Verification items for the finished model (mm, model axes). Round coordinates to 2 decimals unless told otherwise and drop trailing zeros. Write each loop counter-clockwise with the first axis right and the second up, starting at its lowest first coordinate (ties: lowest second). Pieces come first, ordered by that corner, then holes. Notation, with made-up numbers: (20, 83.25) -> (26, 83.25) arc R20 ccw to (26, 122.25) -> close; hole circle Ø11 at (62.25, 46.5). An arc over 180 degrees is marked (long way). Use CSV: the item, a comma, the result in double quotes.
```python
from build123d import *

# Parameters (mm, degrees)
SKETCH1_W           = 40
SKETCH1_H           = 5
BOSS_EXTRUDE1_DEPTH = 72
SKETCH2_W           = 8
SKETCH2_H           = 72
CUT_EXTRUDE1_DEPTH  = 0.75
SKETCH3_W           = 0.6
SKETCH3_H           = 0.6
BOSS_EXTRUDE2_DEPTH = 8
SKETCH4_R           = 2.6
CUT_EXTRUDE2_DEPTH  = 83.516664984
SKETCH5_W           = 8
SKETCH5_H           = 20
CUT_EXTRUDE3_DEPTH  = 83.516664984


with BuildPart() as part:
    # Sketch1 → Boss-Extrude1 (new body)
    with BuildSketch(Plane(origin=(0, 0, 0), x_dir=(1, 0, 0), z_dir=(0, 1, 0))):
        with Locations((20, 2.5)):
            Rectangle(SKETCH1_W, SKETCH1_H)
    extrude(amount=BOSS_EXTRUDE1_DEPTH)

    # Sketch2 → Cut-Extrude1 (cut)
    with BuildSketch(Plane(origin=(0, 0, -5), x_dir=(-1, 0, 0), z_dir=(0, 0, -1))):
        with Locations((-17.2, 36)):
            Rectangle(SKETCH2_W, SKETCH2_H)
    extrude(amount=-CUT_EXTRUDE1_DEPTH, mode=Mode.SUBTRACT)

    # Sketch3 → Boss-Extrude2 (add)
    with BuildSketch(Plane(origin=(13.2, 0, 0), x_dir=(0, 0, -1), z_dir=(1, 0, 0))):
        with Locations((4.55, 71.1)):
            Rectangle(SKETCH3_W, SKETCH3_H)
        with Locations((4.55, 69.1)):
            Rectangle(SKETCH3_W, SKETCH3_H)
        with Locations((4.55, 67.1)):
            Rectangle(SKETCH3_W, SKETCH3_H)
        with Locations((4.55, 65.1)):
            Rectangle(SKETCH3_W, SKETCH3_H)
        with Locations((4.55, 63.1)):
            Rectangle(SKETCH3_W, SKETCH3_H)
        with Locations((4.55, 61.1)):
            Rectangle(SKETCH3_W, SKETCH3_H)
        with Locations((4.55, 59.1)):
            Rectangle(SKETCH3_W, SKETCH3_H)
        with Locations((4.55, 57.1)):
            Rectangle(SKETCH3_W, SKETCH3_H)
        with Locations((4.55, 55.1)):
            Rectangle(SKETCH3_W, SKETCH3_H)
        with Locations((4.55, 53.1)):
            Rectangle(SKETCH3_W, SKETCH3_H)
        with Locations((4.55, 51.1)):
            Rectangle(SKETCH3_W, SKETCH3_H)
        with Locations((4.55, 49.1)):
            Rectangle(SKETCH3_W, SKETCH3_H)
        with Locations((4.55, 47.1)):
            Rectangle(SKETCH3_W, SKETCH3_H)
        with Locations((4.55, 45.1)):
            Rectangle(SKETCH3_W, SKETCH3_H)
        with Locations((4.55, 43.1)):
            Rectangle(SKETCH3_W, SKETCH3_H)
        with Locations((4.55, 41.1)):
            Rectangle(SKETCH3_W, SKETCH3_H)
        with Locations((4.55, 39.1)):
            Rectangle(SKETCH3_W, SKETCH3_H)
        with Locations((4.55, 37.1)):
            Rectangle(SKETCH3_W, SKETCH3_H)
        with Locations((4.55, 35.1)):
            Rectangle(SKETCH3_W, SKETCH3_H)
        with Locations((4.55, 33.1)):
            Rectangle(SKETCH3_W, SKETCH3_H)
        with Locations((4.55, 31.1)):
            Rectangle(SKETCH3_W, SKETCH3_H)
        with Locations((4.55, 29.1)):
            Rectangle(SKETCH3_W, SKETCH3_H)
        with Locations((4.55, 27.1)):
            Rectangle(SKETCH3_W, SKETCH3_H)
        with Locations((4.55, 25.1)):
            Rectangle(SKETCH3_W, SKETCH3_H)
        with Locations((4.55, 23.1)):
            Rectangle(SKETCH3_W, SKETCH3_H)
        with Locations((4.55, 21.1)):
            Rectangle(SKETCH3_W, SKETCH3_H)
        with Locations((4.55, 19.1)):
            Rectangle(SKETCH3_W, SKETCH3_H)
        with Locations((4.55, 17.1)):
            Rectangle(SKETCH3_W, SKETCH3_H)
        with Locations((4.55, 15.1)):
            Rectangle(SKETCH3_W, SKETCH3_H)
        with Locations((4.55, 13.1)):
            Rectangle(SKETCH3_W, SKETCH3_H)
        with Locations((4.55, 11.1)):
            Rectangle(SKETCH3_W, SKETCH3_H)
        with Locations((4.55, 9.1)):
            Rectangle(SKETCH3_W, SKETCH3_H)
        with Locations((4.55, 7.1)):
            Rectangle(SKETCH3_W, SKETCH3_H)
        with Locations((4.55, 5.1)):
            Rectangle(SKETCH3_W, SKETCH3_H)
        with Locations((4.55, 3.1)):
            Rectangle(SKETCH3_W, SKETCH3_H)
        with Locations((4.55, 1.1)):
            Rectangle(SKETCH3_W, SKETCH3_H)
    extrude(amount=BOSS_EXTRUDE2_DEPTH)

    # Sketch4 → Cut-Extrude2 (cut, through all)
    with BuildSketch(Plane.XY):
        with Locations((5, 67)):
            Circle(SKETCH4_R)
        with Locations((35, 67)):
            Circle(SKETCH4_R)
        with Locations((5, 5)):
            Circle(SKETCH4_R)
        with Locations((35, 5)):
            Circle(SKETCH4_R)
        with Locations((5, 36)):
            Circle(SKETCH4_R)
    extrude(amount=-CUT_EXTRUDE2_DEPTH, mode=Mode.SUBTRACT)

    # Sketch5 → Cut-Extrude3 (cut, through all)
    with BuildSketch(Plane.XY):
        with Locations((17.2, 36)):
            Rectangle(SKETCH5_W, SKETCH5_H)
    extrude(amount=-CUT_EXTRUDE3_DEPTH, mode=Mode.SUBTRACT)


solid = part.part
```
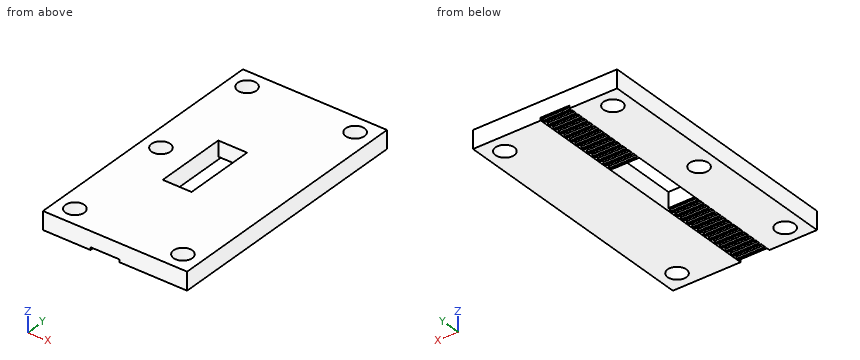
Q1. Section check D-D (y = 36). Record the cut outline in (x, z), plus the area to 3 significant figures.
Filled in:
outline,"(0, -5) -> (2.4, -5) -> (2.4, 0) -> (0, 0) -> close; (7.6, -5) -> (13.2, -5) -> (13.2, 0) -> (7.6, 0) -> close; (21.2, -5) -> (40, -5) -> (40, 0) -> (21.2, 0) -> close"
area,"134 mm²"
Q2. Section check A-A (x = 5). Record the cut outline in (y, z).
Filled in:
outline,"(0, -5) -> (2.4, -5) -> (2.4, 0) -> (0, 0) -> close; (7.6, -5) -> (33.4, -5) -> (33.4, 0) -> (7.6, 0) -> close; (38.6, -5) -> (64.4, -5) -> (64.4, 0) -> (38.6, 0) -> close; (69.6, -5) -> (72, -5) -> (72, 0) -> (69.6, 0) -> close"
Q3. Go/stop test with flat-tipped pins: P1, Ø0.7, axis at x = 17.5, z = -4.5, coming from the +Y side; P2, Ø0.7, axis at x = 17, y = 23, coming from the -Z side; P3, Ø0.7, axis at x = 15.5, y = 56, coming from the -Z side. Record where each tip stops, or that it passes through.
Filled in:
P1,"y = 72"
P2,"z = -4.85"
P3,"z = -4.25"
Q4. Material ranges on L1, parallel to Y at x = 5, z = -2.2; L2, parallel to Y at x = 35, z = -3.05; L3, parallel to Y at x = 16, z = -1.8, recorded low to high.
Filled in:
L1,"0 to 2.4, 7.6 to 33.4, 38.6 to 64.4, 69.6 to 72"
L2,"0 to 2.4, 7.6 to 64.4, 69.6 to 72"
L3,"0 to 26, 46 to 72"
Q5. Section check C-C (x = 36). Record the cut outline in (y, z).
Filled in:
outline,"(0, -5) -> (2.6, -5) -> (2.6, 0) -> (0, 0) -> close; (7.4, -5) -> (64.6, -5) -> (64.6, 0) -> (7.4, 0) -> close; (69.4, -5) -> (72, -5) -> (72, 0) -> (69.4, 0) -> close"
Q6. Section check B-B (y = 44.5). Record the cut outline in (x, z), plus the area to 3 significant figures.
Filled in:
outline,"(0, -5) -> (13.2, -5) -> (13.2, 0) -> (0, 0) -> close; (21.2, -5) -> (40, -5) -> (40, 0) -> (21.2, 0) -> close"
area,"160 mm²"
